The listing builds one solid part. Answer for the finished solid, in the listing's coordinates (mm). Face numbers are marked on the shaded views. Round coordinates to 2 decimals unless told otherwise and drop trailing zeros. Write each loop counter-clockwise with the first axis right and the second up, starting at its lowest first coordinate (ties: lowest second). Pieces come first, ordered by that corner, then holes. Notation, with made-up numbers: M 68,-26.75 L 108,-26.75 A6 cw 108,-21.75 Z; hole C -1.5,15.25 d1. An arc over 180 degrees is marked long. Put each result on its own line as item: value. Start each with the question number.
```python
from build123d import *

# Parameters (mm, degrees)
SKETCH_1_R      = 10
SKETCH_1_R_2    = 5
EXTRUDE_1_DEPTH = 75
SKETCH_2_R      = 12.5
SKETCH_2_R_2    = 7.5
EXTRUDE_2_DEPTH = 10


with BuildPart() as part:
    # 스케치1 → 보스-돌출1 (new, symmetric)
    with BuildSketch(Plane(origin=(0, 0, 0), x_dir=(1, 0, 0), z_dir=(0, 1, 0))):
        with Locations(Location((0, 0, 0), (0, 0, 270))):
            Circle(SKETCH_1_R)
        with Locations(Location((0, 0, 0), (0, 0, 270))):
            Circle(SKETCH_1_R_2, mode=Mode.SUBTRACT)
    extrude(amount=EXTRUDE_1_DEPTH, both=True)

    # 스케치2 → 보스-돌출2 (add, symmetric)
    with BuildSketch(Plane.XY):
        with Locations((0, 82.5)):
            Circle(SKETCH_2_R)
        with Locations((0, 82.5)):
            Circle(SKETCH_2_R_2, mode=Mode.SUBTRACT)
    extrude(amount=EXTRUDE_2_DEPTH, both=True)


solid = part.part
```
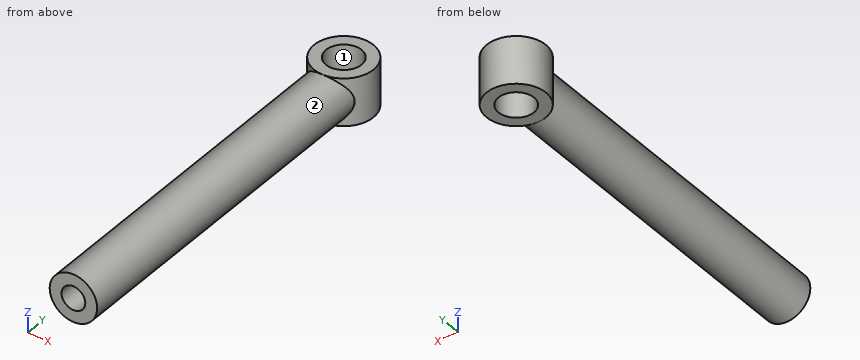
Item 1: Flat-ended cylindrical pins translate along their axes: pin 1 (5 mm diameter, centred on x = -9, z = 1, fed in from +Y); pin 2 (3 mm diameter, centred on x = -7, y = -52.5, fed in from -Z); pin 3 (10 mm diameter, centred on y = -33.5, z = -2.5, fed in from -X). Find the tip coordinate at first contact, or state that the pin passes through.
Item 2: Determine the mould class of the marked faces 1 and 2 for opening direction Y: released by +Y, released by -Y, zero draft, split by the parting line, or undercut.
Item 3: Section C-C (y = 7.5) is taken. Give the vertices of the cut face in (x, z), and give its area (3 significant figures).
Item 4: Section A-A (y = 82.5) is taken. Give the vertices of the cut face in (x, z), and give its area (3 significant figures).
Item 5: Consider line 1 along X through (y, z) = (-36, 0); line 2 along X through (y, z) = (82.5, 0). Determine where each line is inside the solid, lowest interval first. Write a range as [from, to].
Output values:
1. pin 1: stops at y = 93.18
1. pin 2: stops at z = -8.35
1. pin 3: stops at x = -10
2. face 1: undercut
2. face 2: zero draft
3. outline: C 0,0 d20; hole C 0,0 d10
3. area: 236 mm^2
4. outline: M -12.5,-10 L -7.5,-10 L -7.5,10 L -12.5,10 Z; M 7.5,-10 L 12.5,-10 L 12.5,10 L 7.5,10 Z
4. area: 200 mm^2
5. line 1: x = [-10, -5], [5, 10]
5. line 2: x = [-12.5, -7.5], [7.5, 12.5]
